Geometry check sheet. Reference: drawing and pictorial views, mm from the part's lowest x, y, z. A direction names the side the tool comes from. Give positions to 0.01 mm unless a question says otherwise; leave off trailing zeros. Order: outer loops, then holes, each group sorted by start corner. A loop starts at its lowest first (then second) coordinate and runs counter-clockwise, first axis right, second up. Notation, with made-up numbers: (48, -17.75) -> (94, -17.75) arc R19 cw to (94, 12.25) -> close; hole circle Ø6 at (79, 18). An arc over 180 degrees is marked (long way). Write each question's results on one line, items separated by ' | '.
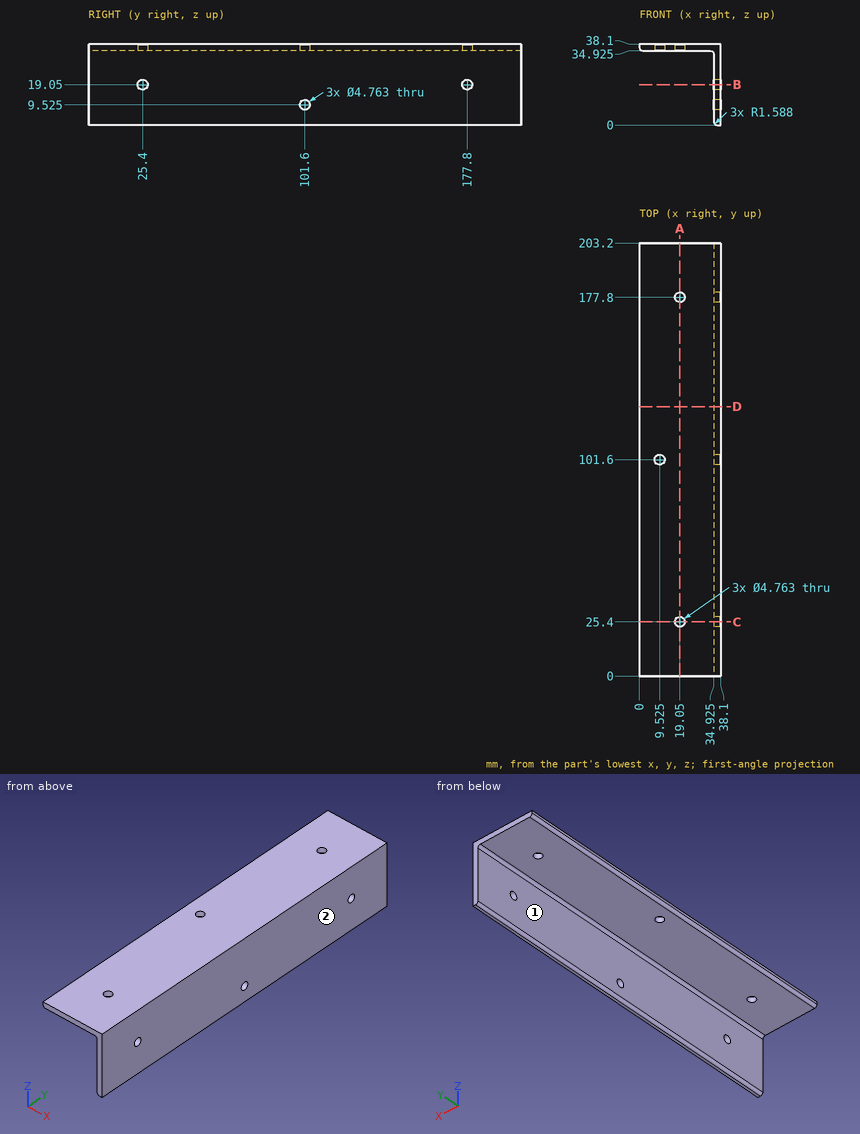
1. Section check B-B on z = 19.05. Record the cut outline in (x, y) (1 decimal), then the cut area to 3 significant figures.
Verdict:
outline: (34.9, 0) -> (38.1, 0) -> (38.1, 23) -> (34.9, 23) -> close; (34.9, 27.8) -> (38.1, 27.8) -> (38.1, 175.4) -> (34.9, 175.4) -> close; (34.9, 180.2) -> (38.1, 180.2) -> (38.1, 203.2) -> (34.9, 203.2) -> close | area: 615 mm^2
2. Access from +Z, -Z, +X, -X, +Y, -Y to the whole of each face (thin tool, end or side, straight path). Record for the marked faces 1 and 2.
Verdict:
face 1: -Z, -X, +Y, -Y | face 2: +Z, -Z, +X, +Y, -Y
3. Material ranges on probe 1 along X at (y, z) = (25.4, 37.25); probe 2 along X at (y, z) = (127.5, 11.5) (1 decimal); probe 3 along Z at (x, y) = (37.4, 101.6), recorded low to high. Write a range as from..to.
Verdict:
probe 1: x = 0..16.67, 21.43..38.1 | probe 2: x = 34.9..38.1 | probe 3: z = 0..7.14, 11.91..38.1
4. Section check C-C on y = 25.4. Record the cut outline in (x, z) (1 decimal).
Verdict:
outline: (0, 36.5) arc R1.6 ccw to (1.6, 34.9) -> (16.7, 34.9) -> (16.7, 38.1) -> (0, 38.1) -> close; (21.4, 34.9) -> (33.3, 34.9) arc R1.6 cw to (34.9, 33.3) -> (34.9, 21.4) -> (38.1, 21.4) -> (38.1, 38.1) -> (21.4, 38.1) -> close; (34.9, 1.6) arc R1.6 ccw to (36.5, 0) -> (38.1, 0) -> (38.1, 16.7) -> (34.9, 16.7) -> close
5. Section check A-A on x = 19.05. Record the cut outline in (y, z) (1 decimal).
Verdict:
outline: (0, 34.9) -> (23, 34.9) -> (23, 38.1) -> (0, 38.1) -> close; (27.8, 34.9) -> (175.4, 34.9) -> (175.4, 38.1) -> (27.8, 38.1) -> close; (180.2, 34.9) -> (203.2, 34.9) -> (203.2, 38.1) -> (180.2, 38.1) -> close
6. Gauge pin test, flat ends, axial feed: pin 1 Ø4 at (y, z) = (177.8, 19.05) entering from +X; pin 2 Ø6 at (y, z) = (25.4, 19.05) entering from -X (1 decimal); pin 3 Ø3 at (x, y) = (11, 121) entering from -Z (1 decimal). Record the tip position at first contact, or that the pin passes through.
Verdict:
pin 1: passes through | pin 2: stops at x = 34.9 | pin 3: stops at z = 34.9
7. Section check D-D on y = 126.5. Record the cut outline in (x, z) (1 decimal), then the cut area to 3 significant figures.
Verdict:
outline: (0, 36.5) arc R1.6 ccw to (1.6, 34.9) -> (33.3, 34.9) arc R1.6 cw to (34.9, 33.3) -> (34.9, 1.6) arc R1.6 ccw to (36.5, 0) -> (38.1, 0) -> (38.1, 38.1) -> (0, 38.1) -> close | area: 231 mm^2
